Build history of the part. All positions in model axes, mm. Give positions to 0.01 mm unless a question says otherwise; leave off trailing zeros. Write each loop counter-clockwise with the first axis right and the second up, starting at its lowest first coordinate (ties: lowest second). Pieces come first, ordered by that corner, then holes. Notation, with made-up numbers: (77, 81.5) -> (113, 81.5) arc R21 cw to (113, 89.5) -> close; hole circle Ø10 at (75, -22). An arc over 180 degrees is marked (long way). Put each result on its own line as item: value.
from build123d import *

# Parameters (mm, degrees)
CROQUIS2_W              = 283
CROQUIS2_H              = 51
SALIENTE_EXTRUIR1_DEPTH = 10
CROQUIS3_R              = 4
CORTAR_EXTRUIR1_DEPTH   = 20
REDONDEO1_R             = 10
REDONDEO2_R             = 10
CORTAR_EXTRUIR4_DEPTH   = 10
REDONDEO3_R             = 15
REDONDEO4_R             = 10


with BuildPart() as part:
    # Croquis2 → Saliente-Extruir1 (new body)
    with BuildSketch(Plane.XY):
        with Locations((141.5, -25.5)):
            Rectangle(CROQUIS2_W, CROQUIS2_H)
    extrude(amount=SALIENTE_EXTRUIR1_DEPTH)

    # Croquis3 → Cortar-Extruir1 (cut)
    with BuildSketch(Plane.XY.offset(10)):
        with Locations((8, -19)):
            Circle(CROQUIS3_R)
        with Locations((54, -19)):
            Circle(CROQUIS3_R)
        with Locations((93, -19)):
            Circle(CROQUIS3_R)
        with Locations((190, -19)):
            Circle(CROQUIS3_R)
        with Locations((229, -19)):
            Circle(CROQUIS3_R)
        with Locations((275, -19)):
            Circle(CROQUIS3_R)
        with BuildLine():
            Line((15, -31), (15, -5))
            Line((15, -5), (47, -5))
            Line((47, -5), (47, -31))
            ThreePointArc((47, -31), (31, -47), (15, -31))
        make_face()
        with BuildLine():
            Line((47.780695143, -41.215325703), (61, -19.5))
            ThreePointArc((61, -19.5), (73.5, -7), (86, -19.5))
            Line((86, -19.5), (98.77233825, -41.15911761))
            ThreePointArc((98.77233825, -41.15911761), (110.619100223, -50.262552209), (125.468650325, -48.616601858))
            Line((125.468650325, -48.616601858), (139.852321867, -40.885601446))
            Line((139.852321867, -40.885601446), (137.350385148, -76.220312807))
            Line((137.350385148, -76.220312807), (73.184426508, -72.914596395))
            Line((73.184426508, -72.914596395), (-5.481789583, -72.914596395))
            Line((-5.481789583, -72.914596395), (-5.481789583, -47.917494117))
            Line((-5.481789583, -47.917494117), (0, -25.5))
            Line((0, -25.5), (16.248287874, -43.974266764))
            ThreePointArc((16.248287874, -43.974266764), (32.712346917, -50.570704554), (47.780695143, -41.215325703))
        make_face()
        with BuildLine():
            Line((100, -31), (100, -5))
            Line((100, -5), (132, -5))
            Line((132, -5), (132, -31))
            ThreePointArc((132, -31), (116, -47), (100, -31))
        make_face()
        with BuildLine():
            Line((143.147678133, -40.885601446), (145.649614852, -76.220312807))
            Line((145.649614852, -76.220312807), (209.815573492, -72.914596395))
            Line((209.815573492, -72.914596395), (288.481789583, -72.914596395))
            Line((288.481789583, -72.914596395), (288.481789583, -47.917494117))
            Line((288.481789583, -47.917494117), (283, -25.5))
            Line((283, -25.5), (266.751712126, -43.974266764))
            ThreePointArc((266.751712126, -43.974266764), (250.287653083, -50.570704554), (235.219304857, -41.215325703))
            Line((235.219304857, -41.215325703), (222, -19.5))
            ThreePointArc((222, -19.5), (209.5, -7), (197, -19.5))
            Line((197, -19.5), (184.22766175, -41.15911761))
            ThreePointArc((184.22766175, -41.15911761), (172.380899777, -50.262552209), (157.531349675, -48.616601858))
            Line((157.531349675, -48.616601858), (143.147678133, -40.885601446))
        make_face()
        with BuildLine():
            Line((151, -5), (151, -31))
            ThreePointArc((151, -31), (167, -47), (183, -31))
            Line((183, -31), (183, -5))
            Line((183, -5), (151, -5))
        make_face()
        with BuildLine():
            Line((236, -5), (236, -31))
            ThreePointArc((236, -31), (252, -47), (268, -31))
            Line((268, -31), (268, -5))
            Line((268, -5), (236, -5))
        make_face()
    extrude(amount=-CORTAR_EXTRUIR1_DEPTH, mode=Mode.SUBTRACT)

    # Redondeo1
    redondeo1_edges = [part.edges().sort_by_distance(p)[0] for p in [
        (61, -19.5, 5),
    ]]
    fillet(redondeo1_edges, radius=REDONDEO1_R)

    # Redondeo2
    redondeo2_edges = [part.edges().sort_by_distance(p)[0] for p in [
        (0, -25.5, 5),
        (86, -19.5, 5),
        (47, -5, 5),
        (15, -5, 5),
        (132, -5, 5),
        (100, -5, 5),
    ]]
    fillet(redondeo2_edges, radius=REDONDEO2_R)

    # Croquis6 → Cortar-Extruir4 (cut)
    with BuildSketch(Plane.XY.offset(10)):
        Polygon((143.147678133, -40.885601446), (141.5, -40), (139.852321867, -40.885601446), (139.136153993, -51), (143.863846007, -51), align=None)
    extrude(amount=-CORTAR_EXTRUIR4_DEPTH, mode=Mode.SUBTRACT)

    # Redondeo3
    redondeo3_edges = [part.edges().sort_by_distance(p)[0] for p in [
        (141.5, -40, 5),
    ]]
    fillet(redondeo3_edges, radius=REDONDEO3_R)

    # Redondeo4
    redondeo4_edges = [part.edges().sort_by_distance(p)[0] for p in [
        (236, -5, 5),
        (268, -5, 5),
        (197, -19.5, 5),
        (222, -19.5, 5),
        (151, -5, 5),
        (183, -5, 5),
    ]]
    fillet(redondeo4_edges, radius=REDONDEO4_R)


solid = part.part
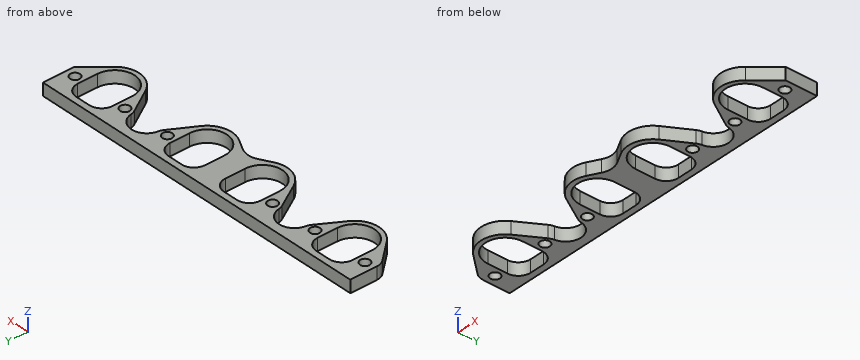
1) Slice it at B-B (y = -11). Write the cut outline in (x, z).
Filled sheet:
outline: (0, 0) -> (15.83, 0) -> (15.83, 10) -> (0, 10) -> close; (46.17, 0) -> (64.33, 0) -> (64.33, 10) -> (46.17, 10) -> close; (82.67, 0) -> (100.83, 0) -> (100.83, 10) -> (82.67, 10) -> close; (131.17, 0) -> (151.83, 0) -> (151.83, 10) -> (131.17, 10) -> close; (182.17, 0) -> (200.33, 0) -> (200.33, 10) -> (182.17, 10) -> close; (218.67, 0) -> (236.83, 0) -> (236.83, 10) -> (218.67, 10) -> close; (267.17, 0) -> (283, 0) -> (283, 10) -> (267.17, 10) -> close
2) Pin check, flat tips, straight feed: pin 1 (5 mm diameter, centred on x = 32, z = 3.5, fed in from -Y); pin 2 (5 mm diameter, centred on x = 127.5, z = 6.5, fed in from -Y). Stop position of each tip, or through.
Filled sheet:
pin 1: y = -50.65
pin 2: y = -48.86
3) Slice it at D-D (z = 5.25). Give the number of separate pieces and of enclosed holes in the cut face, plus the area to 3 significant figures.
Filled sheet:
separate pieces: 1
enclosed holes: 10
area: 5,200 mm2
4) Slice it at A-A (x = 31). Write the cut outline in (y, z).
Filled sheet:
outline: (-50.65, 0) -> (-47, 0) -> (-47, 10) -> (-50.65, 10) -> close; (-5, 0) -> (0, 0) -> (0, 10) -> (-5, 10) -> close
5) Wall check: L1, parallel to Y at x = 229, z = 3.25; L2, parallel to Y at x = 275, z = 2.75; L3, parallel to X at y = -49, z = 3. Give the ranges that are in metal, low to high.
Filled sheet:
L1: -31 to -23, -15 to 0
L2: -34.6 to -23, -15 to 0
L3: 23.13 to 38.87, 107.28 to 124.72, 158.28 to 175.72, 244.13 to 259.87
6) Slice it at C-C (x = 116). Write the cut outline in (y, z), plus the area to 3 significant figures.
Filled sheet:
outline: (-51, 0) -> (-47, 0) -> (-47, 10) -> (-51, 10) -> close; (-5, 0) -> (0, 0) -> (0, 10) -> (-5, 10) -> close
area: 90.0 mm2
